Here's how the part is built. I have some questions about the finished solid (model axes, mm). Face numbers are marked on the shaded views. A direction names the side the tool comes from. Coordinates: 2 decimals unless noted, no trailing zeros. Write each loop counter-clockwise with the first axis right and the second up, starting at its lowest first coordinate (ties: lowest second). Pieces come first, ordered by that corner, then holes.
Item 1: For the marked faces 4 and 5, which set-ups out of +Z, -Z, +X, -X, +Y, -Y let a thin tool reach every point of the face, with its end or its side?
Item 2: I want a section at B-B (z = 191). Please give me the cut outline in (x, y).
Item 3: I want a section at C-C (x = 26.5). Please give me the cut outline in (y, z).
Item 4: If we mould it in two halves opening along X, with no side actions, what happens to the marked faces 1, 2 and 3? For each: pulls with the +X half, pulls with the -X half, needs draft (parallel to the pull), parting line crosses it, or undercut.
Item 5: I'm going to push flat-ended pins straight in: P1, Ø1.9, axis at x = 64.5, z = 156, coming from the -Y side; P2, Ø6, axis at x = 19.5, z = 198.5, coming from the +Y side. Where does each tip first touch, or does it pass through?
Item 6: Please list where these lines run through material, in increasing order: line 1 (X direction, y = 8, z = 228.5); line 2 (Y direction, x = 20.5, z = 203.5).
Item 7: I want a section at D-D (z = 245). Please give me the cut outline in (x, y).
Item 8: I want a section at A-A (y = 9.25). Please give me the cut outline in (x, z), and give its area (3 significant figures).
from build123d import *

# Parameters (mm, degrees)
BASE_FLANGE1_DEPTH = 274.6375
SKETCH2_W          = 91.44
SKETCH2_H          = 127
CUT_EXTRUDE1_DEPTH = 19.05
FILLET1_R          = 4.7625


# Sheet-metal steps are written as plain solids
with BuildPart() as part:
    # Sketch1 → Base-Flange1 (new body)
    with BuildSketch(Plane.XY):
        with BuildLine():
            Line((0, 25.4), (0, 0.7366))
            ThreePointArc((0, 0.7366), (0.215745145, 0.215745145), (0.7366, 0))
            Line((0.7366, 0), (62.7634, 0))
            ThreePointArc((62.7634, 0), (63.284254855, 0.215745145), (63.5, 0.7366))
            Line((63.5, 0.7366), (63.5, 25.4))
            Line((63.5, 25.4), (65.88125, 25.4))
            Line((65.88125, 25.4), (65.88125, 0.7366))
            ThreePointArc((65.88125, 0.7366), (64.968052878, -1.468052878), (62.7634, -2.38125))
            Line((62.7634, -2.38125), (0.7366, -2.38125))
            ThreePointArc((0.7366, -2.38125), (-1.468052878, -1.468052878), (-2.38125, 0.7366))
            Line((-2.38125, 0.7366), (-2.38125, 25.4))
            Line((-2.38125, 25.4), (0, 25.4))
        make_face()
    extrude(amount=BASE_FLANGE1_DEPTH)

    # Sketch2 → Cut-Extrude1 (cut)
    with BuildSketch(Plane.XZ.offset(2.38125)):
        with Locations((31.75, 137.31875)):
            Rectangle(SKETCH2_W, SKETCH2_H)
    extrude(amount=-CUT_EXTRUDE1_DEPTH, mode=Mode.SUBTRACT)

    # Fillet1
    fillet1_edges = [part.edges().sort_by_distance(p)[0] for p in [
        (-1.190625, 16.66875, 73.81875),
        (64.690625, 16.66875, 73.81875),
        (64.690625, 16.66875, 200.81875),
        (-1.190625, 16.66875, 200.81875),
    ]]
    fillet(fillet1_edges, radius=FILLET1_R)


solid = part.part
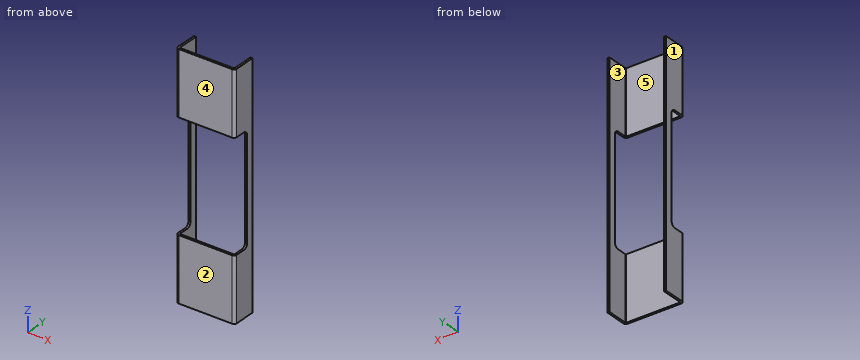
Answer:
1. face 4: +Z, -Z, +X, -X, -Y
1. face 5: +Z, -Z, +Y
2. outline: (-2.38, 16.67) - (0, 16.67) - (0, 25.4) - (-2.38, 25.4) - close; (63.5, 16.67) - (65.88, 16.67) - (65.88, 25.4) - (63.5, 25.4) - close
3. outline: (-2.38, 0) - (0, 0) - (0, 73.82) - (-2.38, 73.82) - close; (-2.38, 200.82) - (0, 200.82) - (0, 274.64) - (-2.38, 274.64) - close
4. face 1: pulls with the -X half
4. face 2: needs draft
4. face 3: undercut
5. P1: stops at y = 16.67
5. P2: stops at y = 0
6. line 1: x = -2.38 to 0, 63.5 to 65.88
6. line 2: y = -2.38 to 0
7. outline: (-2.38, 0.74) arc R3.12 ccw to (0.74, -2.38) - (62.76, -2.38) arc R3.12 ccw to (65.88, 0.74) - (65.88, 25.4) - (63.5, 25.4) - (63.5, 0.74) arc R0.74 cw to (62.76, 0) - (0.74, 0) arc R0.74 cw to (0, 0.74) - (0, 25.4) - (-2.38, 25.4) - close
8. outline: (-2.38, 0) - (0, 0) - (0, 73.82) - (-2.38, 73.82) - close; (-2.38, 200.82) - (0, 200.82) - (0, 274.64) - (-2.38, 274.64) - close; (63.5, 0) - (65.88, 0) - (65.88, 73.82) - (63.5, 73.82) - close; (63.5, 200.82) - (65.88, 200.82) - (65.88, 274.64) - (63.5, 274.64) - close
8. area: 703 mm2
